Design review of the part built by this model. Coordinates are the model's own, in mm. A direction names the side the tool comes from. Coordinates: 2 decimals unless noted, no trailing zeros. Write each loop counter-clockwise with the first axis right and the second up, starting at its lowest first coordinate (ties: lowest second). Pieces come first, ordered by that corner, then holes.
Q1. Take a section at B-B, the plane z = -2.25. Write out the cut boundary in (x, y).
Q2. The part is to be moulded in two halves that separate along Z. For faces 1 (the flat face through (-21, 14, 1.5)), 2 (the flat face through (-21, 2, 0)), 3 (the flat face through (-23.033, 3, 3)), say which applies: released by +Z, released by -Z, zero draft, split by the parting line, or undercut.
Q3. Take a section at D-D, the plane z = -4.7. Write out the cut boundary in (x, y), plus the area to 3 significant figures.
Q4. For L1, parallel to X at y = 2.5, z = 3.75; L2, parallel to Z at x = -27, y = 12.5; L3, parallel to Y at x = -36, z = -3, list the stretches that pass through material, from the lowest coordinate up.
Q5. Take a section at A-A, the plane y = 5.25. Write out the cut boundary in (x, z), plus the area to 3 significant figures.
Q6. For faces 4 (the flat face through (-29.816, 11.025, 3.127)), 5 (the flat face through (-30.112, 5.295, 3.053)), 6 (the flat face through (-12.354, 11.198, 3.042)), 7 (the flat face through (-29.922, 11.216, 3.042)), list the 3-axis set-ups (+Z, -Z, +X, -X, +Y, -Y) from which the entire face can be reached by the end or side of a thin tool; tool diameter is ignored.
Q7. For pin 1 Ø3 at (x, y) = (-21.5, 13.5) entering from +Z; pin 2 Ø5 at (x, z) = (-30, 1.5) entering from -Y; pin 3 Ø1 at (x, z) = (-12.5, 1) entering from +Y, all flat-tipped, find the tip position at first contact; note any pin that passes through.
Q8. Take a section at C-C, the plane x = -26.5. Write out the cut boundary in (y, z).
from build123d import *

# Parameters (mm, degrees)
BOSS_EXTRUDE3_DEPTH      = 4
CUT_EXTRUDE1_DEPTH       = 2.5
BOSS_EXTRUDE4_DEPTH      = 16
BOSS_EXTRUDE4_DEPTH_BACK = 20


with BuildPart() as part:
    # Sketch1 → Boss-Extrude3 (new body)
    with BuildSketch(Plane.XY):
        with BuildLine():
            Line((-23.233269255, 11.836996221), (-36.801095313, 10.577126659))
            ThreePointArc((-36.801095313, 10.577126659), (-39.121917966, 8.246850113), (-36.801095313, 5.916573567))
            Line((-36.801095313, 5.916573567), (-23.233269255, 4.656704004))
            Line((-23.233269255, 4.656704004), (-23.233269255, 1.896850113))
            ThreePointArc((-23.233269255, 1.896850113), (-21.233269255, -0.103149887), (-19.233269255, 1.896850113))
            Line((-19.233269255, 1.896850113), (-19.233269255, 4.656704004))
            Line((-19.233269255, 4.656704004), (-5.665443198, 5.916573567))
            ThreePointArc((-5.665443198, 5.916573567), (-3.344620545, 8.246850113), (-5.665443198, 10.577126659))
            Line((-5.665443198, 10.577126659), (-19.233269255, 11.836996221))
            Line((-19.233269255, 11.836996221), (-19.233269255, 14.596850113))
            ThreePointArc((-19.233269255, 14.596850113), (-21.233269255, 16.596850113), (-23.233269255, 14.596850113))
            Line((-23.233269255, 14.596850113), (-23.233269255, 11.836996221))
        make_face()
    extrude(amount=BOSS_EXTRUDE3_DEPTH)

    # Sketch4 → Cut-Extrude1 (cut)
    with BuildSketch(Plane.XY.offset(4)):
        with BuildLine():
            Line((-23.033269255, 11.654707255), (-36.791622165, 10.377145914))
            ThreePointArc((-36.791622165, 10.377145914), (-38.921917966, 8.246850113), (-36.791622165, 6.116554311))
            Line((-36.791622165, 6.116554311), (-23.033269255, 4.83899297))
            Line((-23.033269255, 4.83899297), (-23.033269255, 1.896850113))
            ThreePointArc((-23.033269255, 1.896850113), (-21.233269255, 0.096850113), (-19.433269255, 1.896850113))
            Line((-19.433269255, 1.896850113), (-19.433269255, 4.83899297))
            Line((-19.433269255, 4.83899297), (-5.674916346, 6.116554311))
            ThreePointArc((-5.674916346, 6.116554311), (-3.544620545, 8.246850113), (-5.674916346, 10.377145914))
            Line((-5.674916346, 10.377145914), (-19.433269255, 11.654707255))
            Line((-19.433269255, 11.654707255), (-19.433269255, 14.596850113))
            ThreePointArc((-19.433269255, 14.596850113), (-21.233269255, 16.396850113), (-23.033269255, 14.596850113))
            Line((-23.033269255, 14.596850113), (-23.033269255, 11.654707255))
        make_face()
    extrude(amount=-CUT_EXTRUDE1_DEPTH, mode=Mode.SUBTRACT)

    # Sketch6 → Boss-Extrude4 (add, two sides)
    with BuildSketch(Plane(origin=(-19.233269255, 0, 0), x_dir=(0, 0, -1), z_dir=(1, 0, 0))) as boss_extrude4_sk:
        with BuildLine():
            ThreePointArc((8.595792289, 10.879439419), (0.000480489, 8.183014626), (8.669380496, 5.733470939))
            ThreePointArc((8.669380496, 5.733470939), (-2.786430444, 8.143161335), (8.595792289, 10.879439419))
        make_face()
    extrude(amount=BOSS_EXTRUDE4_DEPTH)
    extrude(boss_extrude4_sk.sketch, amount=-BOSS_EXTRUDE4_DEPTH_BACK)


solid = part.part
Responses:
1. outline: (-39.23, 2.31) - (-3.23, 2.31) - (-3.23, 4.24) - (-39.23, 4.24) - close; (-39.23, 12.26) - (-3.23, 12.26) - (-3.23, 14.15) - (-39.23, 14.15) - close
2. face 1: released by +Z
2. face 2: undercut
2. face 3: zero draft
3. outline: (-39.23, 2.42) - (-3.23, 2.42) - (-3.23, 3.55) - (-39.23, 3.55) - close; (-39.23, 12.95) - (-3.23, 12.95) - (-3.23, 14.04) - (-39.23, 14.04) - close
3. area: 80.1 mm2
4. L1: x = -23.23 to -23.03, -19.43 to -19.23
4. L2: z = -7.43 to -6.71, -2.69 to 1
4. L3: y = 2.23 to 3.87, 12.63 to 14.23
5. outline: (-39.23, -8.42) - (-3.23, -8.42) - (-3.23, -8.32) - (-39.23, -8.32) - close; (-39.23, -1.08) - (-3.23, -1.08) - (-3.23, 2) - (-12.84, 2) - (-12.84, 4) - (-15.01, 4) - (-15.01, 2) - (-27.46, 2) - (-27.46, 4) - (-29.62, 4) - (-29.62, 2) - (-39.23, 2) - close
5. area: 123 mm2
6. face 4: +Z
6. face 5: +Z, -X, -Y
6. face 6: +Z, +X, +Y
6. face 7: +Z, -X, +Y
7. pin 1: stops at z = 1.5
7. pin 2: stops at y = 2.65
7. pin 3: stops at y = 12.94
8. outline: (4.96, 1.82) arc R6 ccw to (5.73, -8.67) arc R4.7 cw (long way) to (10.88, -8.6) arc R6 ccw to (11.53, 1.79) - (11.53, 4) - (11.33, 4) - (11.33, 1.92) arc R6 ccw to (5.16, 1.94) - (5.16, 4) - (4.96, 4) - close
